```python
from build123d import *

# Parameters (mm, degrees)
SKETCH_1_R      = 0.82794133
SKETCH_1_R_2    = 1
SKETCH_1_R_3    = 0.3
EXTRUDE_3_DEPTH = 50


with BuildPart() as part:
    # 草图1 → 凸台-拉伸3 (new body)
    with BuildSketch(Plane.XY):
        Polygon((20.69853326, 0), (0, 0), (0, -24.135547841), (31.04779989, -24.135547841), (42.400668091, -12.081204645), align=None)
        with Locations((20.69853326, -12.081204645)):
            Circle(SKETCH_1_R, mode=Mode.SUBTRACT)
        with Locations((33.43169801, -17.796901608)):
            Circle(SKETCH_1_R_2, mode=Mode.SUBTRACT)
        with Locations((20.69853326, -3)):
            Circle(SKETCH_1_R, mode=Mode.SUBTRACT)
        with Locations((33.43169801, -17.796901608)):
            Circle(SKETCH_1_R_2)
        with Locations((33.43169801, -17.796901608)):
            Circle(SKETCH_1_R_3, mode=Mode.SUBTRACT)
        with Locations((20.69853326, -12.081204645)):
            Circle(SKETCH_1_R)
        with Locations((20.69853326, -12.081204645)):
            Circle(SKETCH_1_R_3, mode=Mode.SUBTRACT)
        with Locations((20.69853326, -3)):
            Circle(SKETCH_1_R)
        with Locations((20.69853326, -3)):
            Circle(SKETCH_1_R_3, mode=Mode.SUBTRACT)
        Polygon((0, 0), (-20.69853326, 0), (-42.400668091, -12.081204645), (-31.04779989, -24.135547841), (0, -24.135547841), align=None)
        with Locations((-33.43169801, -17.796901608)):
            Circle(SKETCH_1_R_2, mode=Mode.SUBTRACT)
        with Locations((-20.69853326, -12.081204645)):
            Circle(SKETCH_1_R, mode=Mode.SUBTRACT)
        with Locations((-20.69853326, -3)):
            Circle(SKETCH_1_R, mode=Mode.SUBTRACT)
        with Locations((-33.43169801, -17.796901608)):
            Circle(SKETCH_1_R_2)
        with Locations((-33.43169801, -17.796901608)):
            Circle(SKETCH_1_R_3, mode=Mode.SUBTRACT)
        with Locations((-20.69853326, -12.081204645)):
            Circle(SKETCH_1_R)
        with Locations((-20.69853326, -12.081204645)):
            Circle(SKETCH_1_R_3, mode=Mode.SUBTRACT)
        with Locations((-20.69853326, -3)):
            Circle(SKETCH_1_R)
        with Locations((-20.69853326, -3)):
            Circle(SKETCH_1_R_3, mode=Mode.SUBTRACT)
    extrude(amount=EXTRUDE_3_DEPTH)


solid = part.part
```
Input: part model. Units: mm. Frame: model coordinates. Give positions to 0.01 mm unless a question says otherwise; leave off trailing zeros. Order: outer loops, then holes, each group sorted by start corner. A loop starts at its lowest first (then second) coordinate and runs counter-clockwise, first axis right, second up. Notation, with made-up numbers: M 54,-4 L 113,-4 A13 cw 113,1 Z; hole C 86.25,17 d8. An arc over 180 degrees is marked long. One line per question, with ' | ' between items. Start each with the question number.
1. Section query B-B (y = -9). Return the cut outline in (x, z), and give its area (3 significant figures).
2. Section query C-C (x = 29.5). Return the cut outline in (y, z).
3. Section query A-A (z = 25.5). Return the cut outline in (x, y), and give its area (3 significant figures).
4. Material intervals for probe 1 along X at (y, z) = (-14, 21); probe 2 along X at (y, z) = (-14.5, 42.5); probe 3 along Y at (x, z) = (-32, 23), sorted ascending. Write a range as [from, to].
5. First-contact query: pin 1 Ø10 at (y, z) = (-3, 20) entering from -X. Flat tip, straight axial feed; report the tip coordinate or a pass-through.
Here are the results:
1) outline: M -36.87,0 L 36.87,0 L 36.87,50 L -36.87,50 Z | area: 3,690 mm²
2) outline: M -24.14,0 L -4.9,0 L -4.9,50 L -24.14,50 Z
3) outline: M -42.4,-12.08 L -31.05,-24.14 L 31.05,-24.14 L 42.4,-12.08 L 20.7,0 L -20.7,0 Z; hole C -33.43,-17.8 d0.6; hole C -20.7,-12.08 d0.6; hole C -20.7,-3 d0.6; hole C 20.7,-12.08 d0.6; hole C 20.7,-3 d0.6; hole C 33.43,-17.8 d0.6 | area: 1,650 mm²
4) probe 1: [-40.59, 40.59] | probe 2: [-40.12, 40.12] | probe 3: [-23.12, -6.29]
5) pin 1: x = -35.07
